from build123d import *

# Parameters (mm, degrees)
F0_R     = 1.905
F1_DEPTH = 3.175
F2_DEPTH = 1.55575
F0_W     = 6.35
F0_H     = 3.175
F3_DEPTH = 32.385
F5_W     = 6.35
F5_H     = 3.175
F6_DEPTH = 3.81
F4_W     = 6.35
F4_H     = 3.175
F7_DEPTH = 3.81


with BuildPart() as f1:
    # F0 (on Top) → F1 (new body)
    with BuildSketch(Plane.XY):
        with BuildLine():
            ThreePointArc((18.7835533113, -3.175), (17.5708112256, 0), (18.7835533113, 3.175))
            Line((18.7835533113, 3.175), (7.2748389157, 3.175))
            ThreePointArc((7.2748389157, 3.175), (7.7700688589, 1.6217077968), (7.9375, 0))
            ThreePointArc((7.9375, 0), (7.7700688589, -1.6217077968), (7.2748389157, -3.175))
            Line((7.2748389157, -3.175), (18.7835533113, -3.175))
        make_face()
        with BuildLine():
            ThreePointArc((18.7835533113, -3.175), (18.9832714591, -1.5930802583), (19.05, 0))
            ThreePointArc((19.05, 0), (18.9832714591, 1.5930802583), (18.7835533113, 3.175))
            ThreePointArc((18.7835533113, 3.175), (17.5708112256, 0), (18.7835533113, -3.175))
        make_face()
        with BuildLine():
            ThreePointArc((18.7835533113, 3.175), (18.9832714591, 1.5930802583), (19.05, 0))
            ThreePointArc((19.05, 0), (18.9832714591, -1.5930802583), (18.7835533113, -3.175))
            ThreePointArc((18.7835533113, -3.175), (24.0326764282, -4.4489958596), (27.0958112256, 0))
            ThreePointArc((27.0958112256, 0), (24.0326764282, 4.4489958596), (18.7835533113, 3.175))
        make_face()
        with Locations((22.3333112256, 0)):
            Circle(F0_R, mode=Mode.SUBTRACT)
        with BuildLine():
            ThreePointArc((-3.175, 7.2748389157), (0, 7.9375), (3.175, 7.2748389157))
            Line((3.175, 7.2748389157), (3.175, 13.97))
            Line((3.175, 13.97), (-3.175, 13.97))
            Line((-3.175, 13.97), (-3.175, 7.2748389157))
        make_face()
        with BuildLine():
            ThreePointArc((7.9375, 0), (7.7700688589, 1.6217077968), (7.2748389157, 3.175))
            ThreePointArc((7.2748389157, 3.175), (5.6126600757, 5.6126600757), (3.175, 7.2748389157))
            ThreePointArc((3.175, 7.2748389157), (0, 7.9375), (-3.175, 7.2748389157))
            ThreePointArc((-3.175, 7.2748389157), (-5.6126600757, 5.6126600757), (-7.2748389157, 3.175))
            ThreePointArc((-7.2748389157, 3.175), (-7.9375, 0), (-7.2748389157, -3.175))
            ThreePointArc((-7.2748389157, -3.175), (-5.6126600757, -5.6126600757), (-3.175, -7.2748389157))
            ThreePointArc((-3.175, -7.2748389157), (0, -7.9375), (3.175, -7.2748389157))
            ThreePointArc((3.175, -7.2748389157), (5.6126600757, -5.6126600757), (7.2748389157, -3.175))
            ThreePointArc((7.2748389157, -3.175), (7.7700688589, -1.6217077968), (7.9375, 0))
        make_face()
        with BuildLine():
            ThreePointArc((3.5921024484, 3.5921024484), (4.6933080252, 1.9440318364), (5.08, 0))
            ThreePointArc((5.08, 0), (-4.6933080252, -1.9440318364), (3.5921024484, 3.5921024484))
        make_face(mode=Mode.SUBTRACT)
        with BuildLine():
            Line((-7.2748389157, 3.175), (-18.7835533113, 3.175))
            ThreePointArc((-18.7835533113, 3.175), (-17.8843153661, 1.6993652025), (-17.5708112256, 0))
            ThreePointArc((-17.5708112256, 0), (-17.8843153661, -1.6993652025), (-18.7835533113, -3.175))
            Line((-18.7835533113, -3.175), (-7.2748389157, -3.175))
            ThreePointArc((-7.2748389157, -3.175), (-7.9375, 0), (-7.2748389157, 3.175))
        make_face()
        with BuildLine():
            Line((3.175, -13.97), (3.175, -7.2748389157))
            ThreePointArc((3.175, -7.2748389157), (0, -7.9375), (-3.175, -7.2748389157))
            Line((-3.175, -7.2748389157), (-3.175, -13.97))
            Line((-3.175, -13.97), (3.175, -13.97))
        make_face()
        with BuildLine():
            ThreePointArc((-17.5708112256, 0), (-17.8843153661, 1.6993652025), (-18.7835533113, 3.175))
            ThreePointArc((-18.7835533113, 3.175), (-19.05, 0), (-18.7835533113, -3.175))
            ThreePointArc((-18.7835533113, -3.175), (-17.8843153661, -1.6993652025), (-17.5708112256, 0))
        make_face()
        with BuildLine():
            ThreePointArc((-18.7835533113, -3.175), (-19.05, 0), (-18.7835533113, 3.175))
            ThreePointArc((-18.7835533113, 3.175), (-27.0958112256, 0), (-18.7835533113, -3.175))
        make_face()
        with Locations((-22.3333112256, 0)):
            Circle(F0_R, mode=Mode.SUBTRACT)
    extrude(amount=F1_DEPTH)



with BuildPart() as f1b:
    # F0 (on Top) → F1, piece 2 (new body)
    with BuildSketch(Plane.XY):
        with BuildLine():
            Line((3.175, 17.145), (3.175, 18.7835533113))
            ThreePointArc((3.175, 18.7835533113), (0, 17.5708112256), (-3.175, 18.7835533113))
            Line((-3.175, 18.7835533113), (-3.175, 17.145))
            Line((-3.175, 17.145), (3.175, 17.145))
        make_face()
        with BuildLine():
            ThreePointArc((-3.175, 18.7835533113), (0, 19.05), (3.175, 18.7835533113))
            ThreePointArc((3.175, 18.7835533113), (4.3475478002, 20.3890287423), (4.7625, 22.3333112256))
            ThreePointArc((4.7625, 22.3333112256), (-1.9442824833, 26.6808590258), (-3.175, 18.7835533113))
        make_face()
        with Locations((0, 22.3333112256)):
            Circle(F0_R, mode=Mode.SUBTRACT)
        with BuildLine():
            ThreePointArc((-3.175, 18.7835533113), (0, 17.5708112256), (3.175, 18.7835533113))
            ThreePointArc((3.175, 18.7835533113), (0, 19.05), (-3.175, 18.7835533113))
        make_face()
    extrude(amount=F1_DEPTH)


with BuildPart() as f1c:
    # F0 (on Top) → F1, piece 3 (new body)
    with BuildSketch(Plane.XY):
        with BuildLine():
            ThreePointArc((-3.175, -18.7835533113), (0, -17.5708112256), (3.175, -18.7835533113))
            Line((3.175, -18.7835533113), (3.175, -17.145))
            Line((3.175, -17.145), (-3.175, -17.145))
            Line((-3.175, -17.145), (-3.175, -18.7835533113))
        make_face()
        with BuildLine():
            ThreePointArc((-3.175, -18.7835533113), (0, -19.05), (3.175, -18.7835533113))
            ThreePointArc((3.175, -18.7835533113), (0, -17.5708112256), (-3.175, -18.7835533113))
        make_face()
        with BuildLine():
            ThreePointArc((4.7625, -22.3333112256), (4.3475478002, -20.3890287423), (3.175, -18.7835533113))
            ThreePointArc((3.175, -18.7835533113), (0, -19.05), (-3.175, -18.7835533113))
            ThreePointArc((-3.175, -18.7835533113), (-1.9442824833, -26.6808590258), (4.7625, -22.3333112256))
        make_face()
        with Locations((0, -22.3333112256)):
            Circle(F0_R, mode=Mode.SUBTRACT)
    extrude(amount=F1_DEPTH)


with BuildPart() as f1_1:
    add(f1.part)

    add(f1b.part)  # F2 merges F1b

    add(f1c.part)  # F2 merges F1c
    # F0 (on Top) → F2 (join)
    with BuildSketch(Plane.XY):
        with BuildLine():
            Line((7.2748389157, 3.175), (18.7835533113, 3.175))
            ThreePointArc((18.7835533113, 3.175), (13.4703841816, 13.4703841816), (3.175, 18.7835533113))
            Line((3.175, 18.7835533113), (3.175, 17.145))
            Line((3.175, 17.145), (3.175, 13.97))
            Line((3.175, 13.97), (3.175, 7.2748389157))
            ThreePointArc((3.175, 7.2748389157), (5.6126600757, 5.6126600757), (7.2748389157, 3.175))
        make_face()
        with BuildLine():
            ThreePointArc((3.175, -18.7835533113), (13.4703841816, -13.4703841816), (18.7835533113, -3.175))
            Line((18.7835533113, -3.175), (7.2748389157, -3.175))
            ThreePointArc((7.2748389157, -3.175), (5.6126600757, -5.6126600757), (3.175, -7.2748389157))
            Line((3.175, -7.2748389157), (3.175, -13.97))
            Line((3.175, -13.97), (3.175, -17.145))
            Line((3.175, -17.145), (3.175, -18.7835533113))
        make_face()
        with BuildLine():
            Line((-3.175, 17.145), (-3.175, 18.7835533113))
            ThreePointArc((-3.175, 18.7835533113), (-13.4703841816, 13.4703841816), (-18.7835533113, 3.175))
            Line((-18.7835533113, 3.175), (-7.2748389157, 3.175))
            ThreePointArc((-7.2748389157, 3.175), (-5.6126600757, 5.6126600757), (-3.175, 7.2748389157))
            Line((-3.175, 7.2748389157), (-3.175, 13.97))
            Line((-3.175, 13.97), (-3.175, 17.145))
        make_face()
        with BuildLine():
            ThreePointArc((-18.7835533113, -3.175), (-13.4703841816, -13.4703841816), (-3.175, -18.7835533113))
            Line((-3.175, -18.7835533113), (-3.175, -17.145))
            Line((-3.175, -17.145), (-3.175, -13.97))
            Line((-3.175, -13.97), (-3.175, -7.2748389157))
            ThreePointArc((-3.175, -7.2748389157), (-5.6126600757, -5.6126600757), (-7.2748389157, -3.175))
            Line((-7.2748389157, -3.175), (-18.7835533113, -3.175))
        make_face()
    extrude(amount=F2_DEPTH)

    # F0 (on Top) → F3 (join)
    with BuildSketch(Plane.XY):
        with Locations((0, -15.5575)):
            Rectangle(F0_W, F0_H)
        with Locations((0, 15.5575)):
            Rectangle(F0_W, F0_H)
    extrude(amount=F3_DEPTH)

    # F5 (on face) → F6 (join)
    with BuildSketch(Plane(origin=(0, -13.97, 0), x_dir=(-1, 0, 0), z_dir=(0, 1, 0))):
        with Locations((0, 30.7975)):
            Rectangle(F5_W, F5_H)
    extrude(amount=F6_DEPTH)

    # F4 (on face) → F7 (join)
    with BuildSketch(Plane.XZ.offset(-13.97)):
        with Locations((0, 30.7975)):
            Rectangle(F4_W, F4_H)
    extrude(amount=F7_DEPTH)


solid = f1_1.part
The listing builds one solid part. Answer for the finished solid, in the listing's coordinates (mm). A direction names the side the tool comes from. Round coordinates to 2 decimals unless told otherwise and drop trailing zeros. Order: outer loops, then holes, each group sorted by start corner. A loop starts at its lowest first (then second) coordinate and runs counter-clockwise, first axis right, second up. Notation, with made-up numbers: M 62.5,18.25 L 106.5,18.25 A22 cw 106.5,43.25 Z; hole C -26,-33.75 d4. An arc over 180 degrees is marked long. Answer in a Markdown table with one row per item. Add a question column.
1) The part is cut by section A-A on x = 0. Determine the outline of the cut face in (y, z) (3 decimals), plus the area to 3 significant figures.
2) The part is cut by section B-B on z = 7.5. Determine the outline of the cut face in (x, y) (3 decimals), plus the area to 3 significant figures.
3) Determine the mould class of faces 4 (the face through (3.175, 14.4, 16.8)), 5 (the face through (2.05, -22.05, 3.175)), 6 (the face through (0, 12, 29.21)) for opening direction Z: pulls with the +Z half, pulls with the -Z half, needs draft (parallel to the pull), parting line crosses it, or undercut.
4) The part is cut by section D-D on y = -6. Determine the outline of the cut face in (x, z) (3 decimals).
5) Consider line 1 along Y through (x, z) = (0, 1.95); line 2 along Y through (x, z) = (2, 31) (3 decimals); line 3 along Z through (x, y) = (16, -3) (3 decimals). Determine where each line is inside the solid, lowest interval first. Write a range as from..to.
6) The part is cut by section C-C on x = -21.5. Determine the outline of the cut face in (y, z) (3 decimals), plus the area to 3 significant figures.
7) Flat-ended cylindrical pins translate along their axes: pin 1 Ø1.3 at (x, z) = (-12.5, 2) entering from +Y; pin 2 Ø6 at (y, z) = (-15, 15.5) entering from +X (3 decimals); pin 3 Ø5 at (x, z) = (1.5, 16.5) entering from +Y (3 decimals). Find the tip coordinate at first contact, or state that the pin passes through.
8) Which of the six approach directions +Z, -Z, +X, -X, +Y, -Y give full straight-line access (tool end or side, diameter ignored) to faces 1 (the face through (0, 10.16, 31)), 2 (the face through (-9, -9, 1.556)), 3 (the face through (3.175, -14.4, 16.8))?
Findings below:
| question | item | result |
|---|---|---|
| 1 | outline | M -27.096,0 L -24.238,0 L -24.238,3.175 L -27.096,3.175 Z; M -20.428,0 L -5.08,0 L -5.08,3.175 L -13.97,3.175 L -13.97,29.21 L -10.16,29.21 L -10.16,32.385 L -17.145,32.385 L -17.145,3.175 L -20.428,3.175 Z; M 5.08,0 L 20.428,0 L 20.428,3.175 L 17.145,3.175 L 17.145,32.385 L 10.16,32.385 L 10.16,29.21 L 13.97,29.21 L 13.97,3.175 L 5.08,3.175 Z; M 24.238,0 L 27.096,0 L 27.096,3.175 L 24.238,3.175 Z |
| 1 | area | 325 mm² |
| 2 | outline | M -3.175,-17.145 L 3.175,-17.145 L 3.175,-13.97 L -3.175,-13.97 Z; M -3.175,13.97 L 3.175,13.97 L 3.175,17.145 L -3.175,17.145 Z |
| 2 | area | 40.3 mm² |
| 3 | face 4 | needs draft |
| 3 | face 5 | pulls with the +Z half |
| 3 | face 6 | undercut |
| 4 | outline | M -18.08,0 L 18.08,0 L 18.08,1.556 L 5.197,1.556 L 5.197,3.175 L -5.197,3.175 L -5.197,1.556 L -18.08,1.556 Z |
| 5 | line 1 | y = -27.1..-24.24, -20.43..-5.08, 5.08..20.43, 24.24..27.1 |
| 5 | line 2 | y = -17.145..-10.16, 10.16..17.145 |
| 5 | line 3 | z = 0..3.175 |
| 6 | outline | M -4.689,0 L -1.713,0 L -1.713,3.175 L -4.689,3.175 Z; M 1.713,0 L 4.689,0 L 4.689,3.175 L 1.713,3.175 Z |
| 6 | area | 18.9 mm² |
| 7 | pin 1 | stops at y = 14.77 |
| 7 | pin 2 | stops at x = 3.175 |
| 7 | pin 3 | stops at y = 17.145 |
| 8 | face 1 | +Z, +X, -X |
| 8 | face 2 | +Z |
| 8 | face 3 | +Z, +X |
